from build123d import *

# Parameters (mm, degrees)
SKETCH014_R   = 5.975
SKETCH014_R_2 = 2.975
PAD007_DEPTH  = 0.6
PAD008_DEPTH  = 1
SKETCH016_W   = 0.8
SKETCH016_H   = 0.7
PAD009_DEPTH  = 0.6


with BuildPart() as part:
    # Sketch014 → Pad007 (new body)
    with BuildSketch(Plane.XY):
        Circle(SKETCH014_R)
        Circle(SKETCH014_R_2, mode=Mode.SUBTRACT)
    extrude(amount=PAD007_DEPTH)

    # Sketch015 → Pad008 (join, symmetric)
    with BuildSketch(Plane.XZ):
        with BuildLine():
            Line((5.825, 0.6), (6.075, 0.6))
            ThreePointArc((6.075, 0.6), (6.244571, 0.6663), (6.324201, 0.830034))
            Line((6.324201, 0.830034), (6.401917, 1.8))
            Line((6.401917, 1.8), (7, 1.752081))
            Line((7, 1.752081), (6.922285, 0.782114))
            ThreePointArc((6.075, 0), (6.65154, 0.225419), (6.922285, 0.782114))
            Line((6.075, 0), (5.825, 0))
            Line((5.825, 0), (5.825, 0.6))
        make_face()
    extrude(amount=PAD008_DEPTH, both=True)

    # Sketch016 (on Face11 of Pad008) → Pad009 (join)
    with BuildSketch(Plane.XY.offset(0.6)):
        with Locations((3, 0)):
            Rectangle(SKETCH016_W, SKETCH016_H)
    extrude(amount=-PAD009_DEPTH)


with BuildPart() as part_1:
    # Body005 placement: moved
    add(part.part.moved(Location((0, 0, 1.75))))


solid = part_1.part
Part model, mm, in its own coordinate system. A direction names the side the tool comes from. Round coordinates to 2 decimals unless told otherwise and drop trailing zeros. Loops run counter-clockwise (first coordinate to the right, second up) from the corner with the lowest first, then second, coordinate; pieces in that order, holes last. Notation, with made-up numbers: (78, 4) - (101, 4) arc R21 ccw to (101, 20) - close; hole circle Ø5 at (60, 89.25). An arc over 180 degrees is marked (long way). Answer as a JSON object with one key per item and string values.
Item 1: Pull direction X, two halves, no side cores. Call faces 1 (the face through (3, 0, 1.75)), 2 (the face through (-2.972, 0.126, 2.046)), 3 (the face through (6.645, -0.014, 1.969)): pulls with the +X half, pulls with the -X half, needs draft (parallel to the pull), parting line crosses it, or undercut.
Output:
{"face 1": "needs draft", "face 2": "undercut", "face 3": "pulls with the +X half"}
Item 2: Band-saw the part on A-A on y = 0. List the corners of the cut face in (x, z) (3 decimals).
Output:
{"outline": "(-5.975, 1.75) - (-2.975, 1.75) - (-2.975, 2.35) - (-5.975, 2.35) - close; (2.6, 1.75) - (6.075, 1.75) arc R0.85 ccw to (6.922, 2.532) - (7, 3.502) - (6.402, 3.55) - (6.324, 2.58) arc R0.25 cw to (6.075, 2.35) - (2.6, 2.35) - close"}
Item 3: Wall check: L1, parallel to Y at x = 0, z = 2.05 (3 decimals); L2, parallel to Z at x = 4.5, y = -3; L3, parallel to Y at x = 6.75, z = 3.2. Give the ranges that are in metal, low to high.
Output:
{"L1": "-5.975 to -2.975, 2.975 to 5.975", "L2": "1.75 to 2.35", "L3": "-1 to 1"}
Item 4: Band-saw the part on C-C on y = -2. List the corners of the cut face in (x, z), plus the area to 3 significant figures.
Output:
{"outline": "(-5.63, 1.75) - (-2.2, 1.75) - (-2.2, 2.35) - (-5.63, 2.35) - close; (2.2, 1.75) - (5.63, 1.75) - (5.63, 2.35) - (2.2, 2.35) - close", "area": "4.11 mm2"}
Item 5: Band-saw the part on B-B on x = 0. List the corners of the cut face in (y, z) (3 decimals).
Output:
{"outline": "(-5.975, 1.75) - (-2.975, 1.75) - (-2.975, 2.35) - (-5.975, 2.35) - close; (2.975, 1.75) - (5.975, 1.75) - (5.975, 2.35) - (2.975, 2.35) - close"}
Item 6: Tool access for faces 4 (the face through (6.6, -1, 2.7)), 5 (the face through (6.6, 1, 2.7)), 6 (the face through (6.96, -0.01, 3.02)): list every direction of +Z, -Z, +X, -X, +Y, -Y with a clear straight run to the whole face (end or side of a thin tool).
Output:
{"face 4": "+Z, -Z, +X, -Y", "face 5": "+Z, -Z, +X, +Y", "face 6": "-Z, +X, +Y, -Y"}
Item 7: Band-saw the part on D-D on x = 5.5. List the corners of the cut face in (y, z).
Output:
{"outline": "(-2.33, 1.75) - (2.33, 1.75) - (2.33, 2.35) - (-2.33, 2.35) - close"}
Item 8: Pin check, flat tips, straight feed: pin 1 (5 mm diameter, centred on x = -3.5, y = 3, fed in from +Z); pin 2 (0.6 mm diameter, centred on x = 6, z = 3, fed in from +Y); pin 3 (0.6 mm diameter, centred on x = 6.5, z = 2.5, fed in from -Y). Stop position of each tip, or through.
Output:
{"pin 1": "z = 2.35", "pin 2": "through", "pin 3": "y = -1"}
